Geometry check sheet. Reference: drawing and pictorial views, mm from the part's lowest x, y, z. Give positions to 0.01 mm unless a question says otherwise; leave off trailing zeros. Order: outer loops, then holes, each group sorted by start corner. A loop starts at its lowest first (then second) coordinate and runs counter-clockwise, first axis right, second up. Notation, with made-up numbers: (49.25, 87) -> (89.25, 87) arc R30 cw to (89.25, 112) -> close; hole circle Ø1 at (84.25, 75). An arc over 180 degrees is marked (long way). Write each question's results on one line, items separated by ' | '. Start each with the question number.
1. Depth check by flat-ended pin: pin 1 Ø5 at (x, z) = (135.5, 4.5) entering from +Y; pin 2 Ø5 at (y, z) = (96.5, 5.5) entering from -X; pin 3 Ø5 at (y, z) = (44, 6) entering from +X. Enter the tip coordinate at first touch or a pass-through.
2. Material ranges on L1, parallel to Y at x = 170, z = 1.5; L2, parallel to X at y = 18, z = 7.75; L3, parallel to Y at x = 161.5, z = 6, recorded low to high. Write a range as from..to.
3. Cross-section at C-C, the plane y = 97. Enter the section's corners in (x, z), then the cut area to 3 significant figures.
4. Cross-section at A-A, the plane x = 175. Enter the section's corners in (y, z), then the cut area to 3 significant figures.
5. Cross-section at B-B, the plane x = 47.5. Enter the section's corners in (y, z), then the cut area to 3 significant figures.
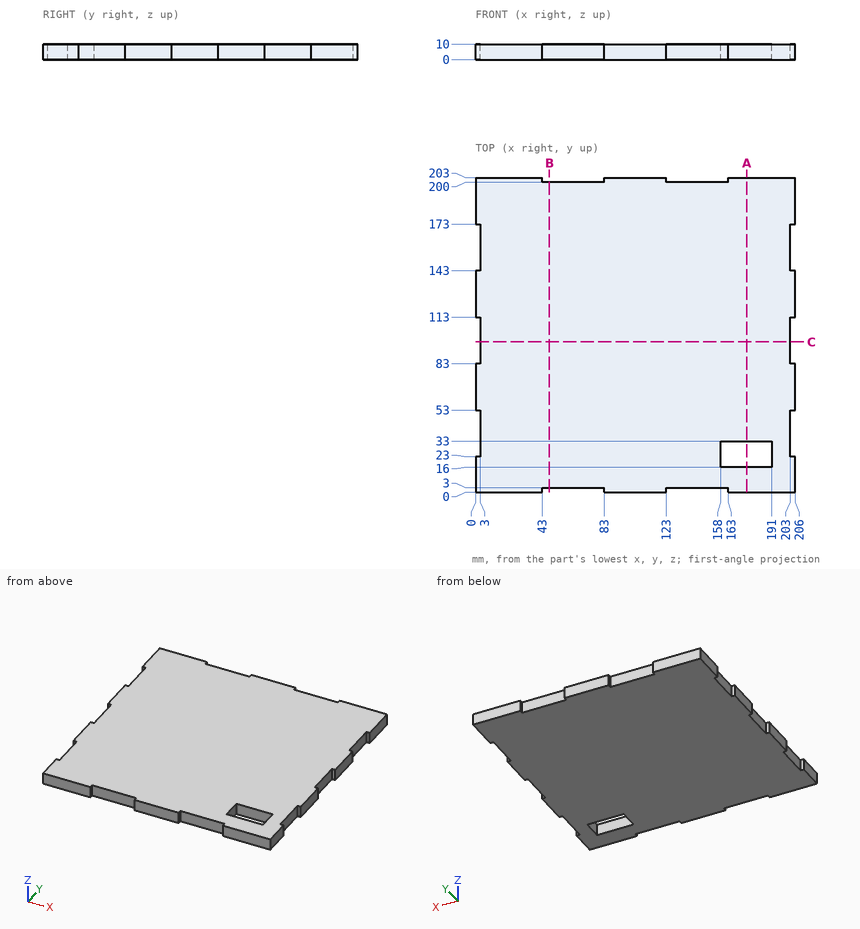
Results below:
1) pin 1: stops at y = 200 | pin 2: stops at x = 3 | pin 3: stops at x = 203
2) L1: y = 0..16, 33..203 | L2: x = 0..158, 191..206 | L3: y = 3..16, 33..200
3) outline: (3, 0) -> (203, 0) -> (203, 10) -> (3, 10) -> close | area: 2,000 mm²
4) outline: (0, 0) -> (16, 0) -> (16, 10) -> (0, 10) -> close; (33, 0) -> (203, 0) -> (203, 10) -> (33, 10) -> close | area: 1,860 mm²
5) outline: (3, 0) -> (200, 0) -> (200, 10) -> (3, 10) -> close | area: 1,970 mm²
